Input: part model. Units: mm. Frame: model coordinates. A direction names the side the tool comes from. Round coordinates to 2 decimals unless told otherwise and drop trailing zeros. Loops run counter-clockwise (first coordinate to the right, second up) from the corner with the lowest first, then second, coordinate; pieces in that order, holes last. Notation, with made-up numbers: (31.25, 21) - (67.25, 21) arc R16 ccw to (67.25, 46) - close; hole circle Ø3 at (-35, 59). An arc over 180 degrees is marked (long way). Use CSV: the item, a comma, the result in double quotes. Start each with the question number.
1. Pin query (flat end, axial travel): P1, Ø12, axis at y = 95, z = 16, coming from the +X side; P2, Ø12, axis at y = 129.5, z = 8.5, coming from the +X side; P3, Ø4, axis at x = 13.5, y = 35.5, coming from the +Z side. Return the tip coordinate at first contact, or that it passes through.
2. Cut plane B-B (x = 20.5). Return loops of the section in (y, z).
3. Pull-direction query (Y, two-part tool) for faces 4 (the flat face through (0, -133, 0)), 5 (the flat face through (-11, 0, 12)), 6 (the flat face through (0, 214, 0)), 7 (the flat face through (0, -17, 25.458)); classes: +Y half, -Y half, draft (parallel to the pull), parting line (faces both ways), or undercut.
4. Material intervals for probe 1 along Y at (x, z) = (19, -12); probe 2 along Y at (x, z) = (-1.5, -7.5); probe 3 along X at (y, z) = (18, -13), sorted ascending. Write a range as from..to.
5. Cut plane C-C (z = 0). Return loops of the section in (x, y), and give its area (3 significant figures).
6. Cut plane D-D (x = 0). Return loops of the section in (y, z), and give its area (3 significant figures).
7. Access query for faces 1 (the flat face through (0, -17, -25.458)), 2 (the cylindrical face through (-0.33, -82.807, -7.493)), 3 (the cylindrical face through (0.66, 88.74, -14.985)). Directions: +Z, -Z, +X, -X, +Y, -Y. A direction counts if a zero-diameter tool reaches every point of the face in a straight line with its end or side. Return the directions, or none.
8. Cut plane A-A (z = -18.5). Return loops of the section in (x, y).
```python
from build123d import *

# Parameters (mm, degrees)
SKETCH1_R           = 15
BOSS_EXTRUDE2_DEPTH = 194
SKETCH2_W           = 50.475671087
SKETCH2_H           = 50.915354634
BOSS_EXTRUDE3_DEPTH = 34
SKETCH3_R           = 7.5
BOSS_EXTRUDE4_DEPTH = 99


with BuildPart() as part:
    # Sketch1 → Boss-Extrude2 (new body)
    with BuildSketch(Plane(origin=(0, 0, 0), x_dir=(1, 0, 0), z_dir=(0, 1, 0))):
        with Locations(Location((0, 0, 0), (0, 0, 270))):
            Circle(SKETCH1_R)
    extrude(amount=BOSS_EXTRUDE2_DEPTH)

    # Sketch2 → Boss-Extrude3 (add)
    with BuildSketch(Plane.XZ):
        with Locations((0.175873419, 0)):
            Rectangle(SKETCH2_W, SKETCH2_H)
    boss_extrude3 = extrude(amount=BOSS_EXTRUDE3_DEPTH)

    # Mirror1: Boss-Extrude3 across plane
    add(boss_extrude3.mirror(Plane.ZX.offset(90)))

    # Sketch3 → Boss-Extrude4 (add)
    with BuildSketch(Plane.XZ.offset(34)):
        with Locations(Location((0, 0, 0), (0, 0, 90))):
            Circle(SKETCH3_R)
    extrude(amount=BOSS_EXTRUDE4_DEPTH)


solid = part.part
```
Established:
1,P1,"stops at x = 11.18"
1,P2,"stops at x = 14.79"
1,P3,"stops at z = 9.63"
2,outline,"(-34, -25.46) - (0, -25.46) - (0, 25.46) - (-34, 25.46) - close; (180, -25.46) - (214, -25.46) - (214, 25.46) - (180, 25.46) - close"
3,face 4,"-Y half"
3,face 5,"undercut"
3,face 6,"+Y half"
3,face 7,"draft"
4,probe 1,"y = -34..0, 180..214"
4,probe 2,"y = -34..214"
4,probe 3,"x = -7.48..7.48"
5,outline,"(-25.06, -34) - (-7.5, -34) - (-7.5, -133) - (7.5, -133) - (7.5, -34) - (25.41, -34) - (25.41, 0) - (15, 0) - (15, 180) - (25.41, 180) - (25.41, 214) - (-25.06, 214) - (-25.06, 180) - (-15, 180) - (-15, 0) - (-25.06, 0) - close"
5,area,"10,300 mm2"
6,outline,"(-133, -7.5) - (-34, -7.5) - (-34, -25.46) - (0, -25.46) - (0, -15) - (180, -15) - (180, -25.46) - (214, -25.46) - (214, 25.46) - (180, 25.46) - (180, 15) - (0, 15) - (0, 25.46) - (-34, 25.46) - (-34, 7.5) - (-133, 7.5) - close"
6,area,"10,300 mm2"
7,face 1,"-Z, +X, -X, +Y, -Y"
7,face 2,"-Y"
7,face 3,"none"
8,outline,"(-25.06, -34) - (25.41, -34) - (25.41, 0) - (-25.06, 0) - close; (-25.06, 180) - (25.41, 180) - (25.41, 214) - (-25.06, 214) - close"
